```python
from build123d import *

# Parameters (mm, degrees)
SMUSSO1_SIZE = 1
SCHIZZO5_W   = 1.6
SCHIZZO5_H   = 4.170885387
SCHIZZO5_W_2 = 0.15


with BuildPart() as part:
    # Schizzo1 → Rivoluzione1 (revolve)
    with BuildSketch(Plane.XY, mode=Mode.PRIVATE) as rivoluzione1_sk:
        Polygon((0, 0), (0, 30), (-20, 30), (-20, 15), (-60, 15), (-60, 0), align=None)
    revolve(rivoluzione1_sk.sketch.rotate(Axis((0, 0, 0), (-1, 0, 0)), 90), axis=Axis((0, 0, 0), (-1, 0, 0)))

    # Smusso1
    smusso1_edges = [part.edges().sort_by_distance(p)[0] for p in [
        (-60, 0, 15),
        (-20, 0, 30),
        (0, 0, 30),
    ]]
    chamfer(smusso1_edges, length=SMUSSO1_SIZE)

    # Schizzo5 → Taglia-Rivoluzione7 (revolve, cut)
    with BuildSketch(Plane.XY, mode=Mode.PRIVATE) as taglia_rivoluzione7_sk:
        with Locations((-50.8, 15.585442694)):
            Rectangle(SCHIZZO5_W, SCHIZZO5_H)
        with Locations((-49.925, 15.585442694)):
            Rectangle(SCHIZZO5_W_2, SCHIZZO5_H)
    revolve(taglia_rivoluzione7_sk.sketch.rotate(Axis((0, 0, 0), (-1, 0, 0)), 270), axis=Axis((0, 0, 0), (-1, 0, 0)), mode=Mode.SUBTRACT)


solid = part.part
```
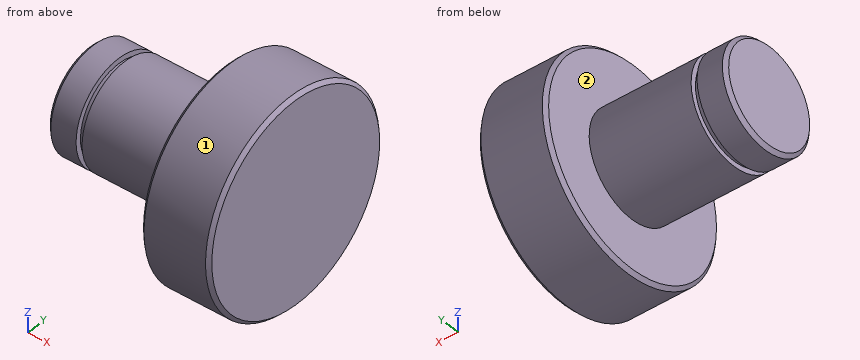
Model file for the job. Use its own axes, mm. Face numbers are marked on the shaded views. A direction names the side the tool comes from. Coordinates: 2 decimals unless noted, no trailing zeros. Write each loop counter-clockwise with the first axis right and the second up, starting at its lowest first coordinate (ties: lowest second). Pieces come first, ordered by that corner, then holes. Notation, with made-up numbers: (-6.75, 46) - (14.25, 46) arc R8 cw to (14.25, 51) - close; hole circle Ø6 at (-22.5, -33.5). An arc over 180 degrees is marked (long way). Use a Markdown table: item, result. Add a question column.
Item 1: Band-saw the part on C-C, the plane x = -18. Write the cut outline in (y, z).
Item 2: Drill centre lines: line 1 along X through (y, z) = (-2, -18); line 2 along Z through (x, y) = (-48, -0.5). Where is each one in solid material? Low to high.
Item 3: Drop flat-ended pins along their axis: pin 1 (2 mm diameter, centred on x = -42.5, z = 10.5, fed in from -Y); pin 2 (5 mm diameter, centred on x = -21.5, z = -18, fed in from -Y); pin 3 (3 mm diameter, centred on x = -25.5, y = 15, fed in from +Z); pin 4 (8 mm diameter, centred on x = -43.5, z = 19.5, fed in from -Y). Give the stop position or say it passes through.
Item 4: Band-saw the part on D-D, the plane x = -33. Write the cut outline in (y, z).
Item 5: 3-axis set-ups, long thin cutter, end or side, ignore diameter. For the marked faces 1 and 2: which of +Z, -Z, +X, -X, +Y, -Y reach the whole face in a straight line?
Item 6: Band-saw the part on A-A, the plane z = 0. Write the cut outline in (x, y), and give its area (3 significant figures).
A:
| question | item | result |
|---|---|---|
| 1 | outline | circle Ø60 at (0, 0) |
| 2 | line 1 | x = -20 to 0 |
| 2 | line 2 | z = -14.99 to 14.99 |
| 3 | pin 1 | stops at y = -11.61 |
| 3 | pin 2 | stops at y = -24.48 |
| 3 | pin 3 | stops at z = 6.54 |
| 3 | pin 4 | passes through |
| 4 | outline | circle Ø30 at (0, 0) |
| 5 | face 1 | +X, -X |
| 5 | face 2 | -X |
| 6 | outline | (-60, -14) - (-59, -15) - (-51.6, -15) - (-51.6, -13.5) - (-49.85, -13.5) - (-49.85, -15) - (-20, -15) - (-20, -29) - (-19, -30) - (-1, -30) - (0, -29) - (0, 29) - (-1, 30) - (-19, 30) - (-20, 29) - (-20, 15) - (-49.85, 15) - (-49.85, 13.5) - (-51.6, 13.5) - (-51.6, 15) - (-59, 15) - (-60, 14) - close |
| 6 | area | 2,390 mm² |
